from build123d import *

# Parameters (mm, degrees)
BOSS_EXTRUDE1_DEPTH = 5
SKETCH2_R           = 2.1
CUT_EXTRUDE1_DEPTH  = 10
BOSS_EXTRUDE2_DEPTH = 5
BOSS_EXTRUDE3_DEPTH = 5
SKETCH5_R           = 2.1
CUT_EXTRUDE2_DEPTH  = 5
BOSS_EXTRUDE4_DEPTH = 5


with BuildPart() as part:
    # Sketch1 → Boss-Extrude1 (new body)
    with BuildSketch(Plane.XY):
        Polygon((-182, 200), (-182, 180), (-187, 180), (-187, 20), (-182, 20), (-182, 0), (0, 0), (0, 20), (5, 20), (5, 180), (0, 180), (0, 200), align=None)
    extrude(amount=BOSS_EXTRUDE1_DEPTH)

    # Sketch2 → Cut-Extrude1 (cut)
    with BuildSketch(Plane(origin=(0, 0, 0), x_dir=(-1, 0, 0), z_dir=(0, 0, -1))):
        with Locations((-2.5, 139.3)):
            Circle(SKETCH2_R)
        with Locations((-2.5, 37.9)):
            Circle(SKETCH2_R)
        with Locations(Location((184.5, 37.9, 0), (0, 0, 180))):
            Circle(SKETCH2_R)
        with Locations(Location((184.5, 139.3, 0), (0, 0, 180))):
            Circle(SKETCH2_R)
    extrude(amount=-CUT_EXTRUDE1_DEPTH, mode=Mode.SUBTRACT)

    # Sketch3 → Boss-Extrude2 (add)
    with BuildSketch(Plane(origin=(0, 0, 0), x_dir=(-1, 0, 0), z_dir=(0, 0, -1))):
        with BuildLine():
            Line((-5, 136.177501001), (-5, 142.422498999))
            ThreePointArc((-5, 142.422498999), (-6.5, 139.3), (-5, 136.177501001))
        make_face()
    boss_extrude2 = extrude(amount=-BOSS_EXTRUDE2_DEPTH)

    # Sketch4 → Boss-Extrude3 (add)
    with BuildSketch(Plane(origin=(0, 0, 0), x_dir=(-1, 0, 0), z_dir=(0, 0, -1))):
        with BuildLine():
            Line((-5, 34.777501001), (-5, 41.022498999))
            ThreePointArc((-5, 41.022498999), (-6.5, 37.9), (-5, 34.777501001))
        make_face()
    boss_extrude3 = extrude(amount=-BOSS_EXTRUDE3_DEPTH)

    # Mirror1: Boss-Extrude2, Boss-Extrude3 across plane
    add(boss_extrude2.mirror(Plane.ZY.offset(91)))
    add(boss_extrude3.mirror(Plane.ZY.offset(91)))

    # Sketch5 → Cut-Extrude2 (cut)
    with BuildSketch(Plane(origin=(0, 0, 0), x_dir=(-1, 0, 0), z_dir=(0, 0, -1))):
        with Locations((30, 2.5)):
            Circle(SKETCH5_R)
        with Locations((152, 2.5)):
            Circle(SKETCH5_R)
    extrude(amount=-CUT_EXTRUDE2_DEPTH, mode=Mode.SUBTRACT)

    # Sketch6 → Boss-Extrude4 (add)
    with BuildSketch(Plane(origin=(0, 0, 0), x_dir=(-1, 0, 0), z_dir=(0, 0, -1))):
        with BuildLine():
            Line((155.122498999, 0), (148.877501001, 0))
            ThreePointArc((148.877501001, 0), (152, -1.5), (155.122498999, 0))
        make_face()
        with BuildLine():
            Line((33.122498999, 0), (26.877501001, 0))
            ThreePointArc((26.877501001, 0), (30, -1.5), (33.122498999, 0))
        make_face()
    extrude(amount=-BOSS_EXTRUDE4_DEPTH)


solid = part.part
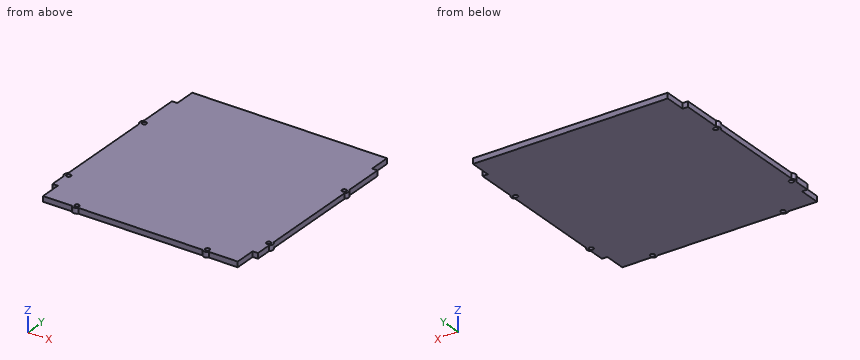
Geometry: final body of the model. Coordinates: model frame, mm. Coordinates: 2 decimals unless noted, no trailing zeros. Loops run counter-clockwise (first coordinate to the right, second up) from the corner with the lowest first, then second, coordinate; pieces in that order, holes last. Notation, with made-up numbers: (63.5, 18.25) - (115.5, 18.25) arc R20 ccw to (115.5, 22.25) - close; hole circle Ø6 at (46.25, 14). An arc over 180 degrees is marked (long way). Put each result on its own line as item: value. Start each with the question number.
Q1. Cut plane A-A, the plane z = 1.3. Give the number of separate pieces and of enclosed holes in the cut face, and give its area (3 significant figures).
Q2. Pin query (flat end, axial travel): pin 1 Ø1.5 at (y, z) = (168.5, 3) entering from -X; pin 2 Ø1.5 at (x, z) = (-75, 3.5) entering from -Y; pin 3 Ø1.5 at (y, z) = (8, 2.5) entering from -X. Return the tip coordinate at first contact, or that it passes through.
Q3. Cut plane B-B, the plane y = 162. Return loops of the section in (x, z).
Q4. Line query: line 1 (Y direction, x = -184.5, z = 2.35); line 2 (X direction, y = 139.3, z = 2.55); line 3 (X direction, y = 165.5, z = 2.55). Output: solid intervals per line, ascending.
Filled sheet:
1. separate pieces: 1
1. enclosed holes: 6
1. area: 38,000 mm²
2. pin 1: x = -187
2. pin 2: y = 0
2. pin 3: x = -182
3. outline: (-187, 0) - (5, 0) - (5, 5) - (-187, 5) - close
4. line 1: 20 to 35.8, 40 to 137.2, 141.4 to 180
4. line 2: -188.5 to -186.6, -182.4 to 0.4, 4.6 to 6.5
4. line 3: -187 to 5
